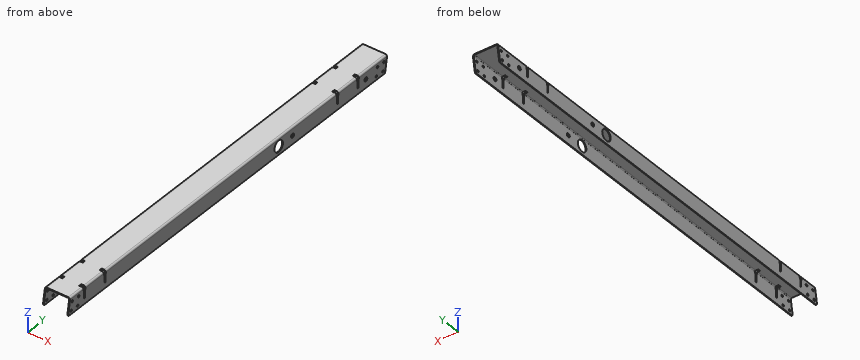
from build123d import *

# Parameters (mm, degrees)
SKETCH1_W                        = 57.15
SKETCH1_H                        = 946.658
BASE_FLANGE1_DEPTH               = 1.89738
EDGE_FLANGE1_STRIP_W             = 11.65352
EDGE_FLANGE1_STRIP_H             = 1.89738
EDGE_FLANGE1_STRIP_CUT_DEPTH     = 946.658
EDGE_FLANGE1_DEPTH               = 946.658
EDGE_FLANGE1_FLAT_DEPTH          = 1.89738
EDGE_FLANGE2_STRIP_W             = 11.65352
EDGE_FLANGE2_STRIP_H             = 1.89738
EDGE_FLANGE2_STRIP_CUT_DEPTH     = 946.658
EDGE_FLANGE2_DEPTH               = 946.658
EDGE_FLANGE2_FLAT_DEPTH          = 1.89738
FILLET1_R                        = 2.54
SKETCH12_R                       = 2.4638
CUT_EXTRUDE1_DEPTH               = 484.620370701
SKETCH13_R                       = 2.4638
CUT_EXTRUDE2_DEPTH               = 484.620370701
CUT_EXTRUDE3_DEPTH               = 9.525
LPATTERN1_COUNT                  = 2
LPATTERN1_PITCH                  = 755.65
MIRROR1_COPY_1_DEPTH             = 9.525
SKETCH15_R                       = 12.7
CUT_EXTRUDE4_DEPTH               = 484.620370701
F_11_32_0_34375_DIAMETER_HOLE1_D = 8.73125


# Sheet-metal steps are written as plain solids
with BuildPart() as part:
    # Sketch1 → Base-Flange1 (new body)
    with BuildSketch(Plane.XY):
        Rectangle(SKETCH1_W, SKETCH1_H)
    extrude(amount=-BASE_FLANGE1_DEPTH)

    # Edge-Flange1 strip (across the edge) → Edge-Flange1 strip cut (cut)
    with BuildSketch(Plane(origin=(28.575, 473.329, -1.89738), x_dir=(-1, 0, 0), z_dir=(0, -1, 0))):
        with Locations((-1.89738, -0.94869)):
            Rectangle(EDGE_FLANGE1_STRIP_W, EDGE_FLANGE1_STRIP_H)
    extrude(amount=EDGE_FLANGE1_STRIP_CUT_DEPTH, mode=Mode.SUBTRACT)

    # Edge-Flange1 bend section (across the edge) → Edge-Flange1 (add)
    with BuildSketch(Plane(origin=(28.575, 473.329, -1.89738), x_dir=(-1, 0, 0), z_dir=(0, -1, 0))):
        with BuildLine():
            Line((0, 2.032), (1.89738, 2.032))
            ThreePointArc((1.89738, 2.032), (2.492539021, 0.595159021), (3.92938, 0))
            Line((3.92938, 0), (3.92938, -1.89738))
            ThreePointArc((3.92938, -1.89738), (1.150888756, -0.746491244), (0, 2.032))
        make_face()
    extrude(amount=EDGE_FLANGE1_DEPTH)

    # Edge-Flange1 profile (on flange) → Edge-Flange1 flat (add)
    with BuildSketch(Plane(origin=(28.575, 0, -1.89738), x_dir=(0, 1, 0), z_dir=(-1, 0, 0))):
        Polygon((473.329, 2.032), (473.329, 2.87782), (467.452938633, 36.20262), (-479.205061367, 36.20262), (-473.329, 2.87782), (-473.329, 2.032), align=None)
    extrude(amount=EDGE_FLANGE1_FLAT_DEPTH)

    # Edge-Flange2 strip (across the edge) → Edge-Flange2 strip cut (cut)
    with BuildSketch(Plane(origin=(-28.575, -473.329, -1.89738), x_dir=(1, 0, 0), z_dir=(0, 1, 0))):
        with Locations((-1.89738, -0.94869)):
            Rectangle(EDGE_FLANGE2_STRIP_W, EDGE_FLANGE2_STRIP_H)
    extrude(amount=EDGE_FLANGE2_STRIP_CUT_DEPTH, mode=Mode.SUBTRACT)

    # Edge-Flange2 bend section (across the edge) → Edge-Flange2 (add)
    with BuildSketch(Plane(origin=(-28.575, -473.329, -1.89738), x_dir=(1, 0, 0), z_dir=(0, 1, 0))):
        with BuildLine():
            Line((0, 2.032), (1.89738, 2.032))
            ThreePointArc((1.89738, 2.032), (2.492539021, 0.595159021), (3.92938, 0))
            Line((3.92938, 0), (3.92938, -1.89738))
            ThreePointArc((3.92938, -1.89738), (1.150888756, -0.746491244), (0, 2.032))
        make_face()
    extrude(amount=EDGE_FLANGE2_DEPTH)

    # Edge-Flange2 profile (on flange) → Edge-Flange2 flat (add)
    with BuildSketch(Plane(origin=(-28.575, 0, -1.89738), x_dir=(0, -1, 0), z_dir=(1, 0, 0))):
        Polygon((-473.329, 2.87782), (-473.329, 2.032), (473.329, 2.032), (473.329, 2.87782), (479.205061367, 36.20262), (-467.452938633, 36.20262), align=None)
    extrude(amount=EDGE_FLANGE2_FLAT_DEPTH)

    # Fillet1
    fillet1_edges = [part.edges().sort_by_distance(p)[0] for p in [
        (27.62631, -479.205061367, -38.1),
        (27.62631, 467.452938633, -38.1),
        (-27.62631, 467.452938633, -38.1),
        (-27.62631, -479.205061367, -38.1),
    ]]
    fillet(fillet1_edges, radius=FILLET1_R)

    # Sketch12 → Cut-Extrude1 (cut, through all)
    with BuildSketch(Plane.ZY.offset(28.575)):
        with Locations((-30.48, -470.123898991)):
            Circle(SKETCH12_R)
        with Locations((-30.48, -450.780022035)):
            Circle(SKETCH12_R)
        with Locations((-11.43, -447.420993052)):
            Circle(SKETCH12_R)
        with Locations((-11.43, -466.764870009)):
            Circle(SKETCH12_R)
    extrude(amount=-CUT_EXTRUDE1_DEPTH, mode=Mode.SUBTRACT)

    # Sketch13 → Cut-Extrude2 (cut, through all)
    with BuildSketch(Plane.ZY.offset(28.575)):
        with Locations((-30.48, 461.058999444)):
            Circle(SKETCH13_R)
        with Locations((-11.43, 464.418028426)):
            Circle(SKETCH13_R)
        with Locations((-11.43, 445.07415147)):
            Circle(SKETCH13_R)
        with Locations((-30.48, 441.715122487)):
            Circle(SKETCH13_R)
    extrude(amount=-CUT_EXTRUDE2_DEPTH, mode=Mode.SUBTRACT)

    # Sketch14 → Cut-Extrude3 (cut)
    with BuildSketch(Plane.ZY.offset(28.575)):
        Polygon((3.175, 389.509), (3.175, 383.159), (-5.08, 383.159), (-10.16, 385.064), (-25.4, 385.064), (-25.4, 387.604), (-10.16, 387.604), (-5.08, 389.509), align=None)
        Polygon((3.175, 328.549), (3.175, 322.199), (-5.08, 322.199), (-10.16, 324.104), (-25.4, 324.104), (-25.4, 326.644), (-10.16, 326.644), (-5.08, 328.549), align=None)
    cut_extrude3 = extrude(amount=-CUT_EXTRUDE3_DEPTH, mode=Mode.SUBTRACT)

    # LPattern1: Cut-Extrude3 ×2
    with Locations(*[(0, -i * LPATTERN1_PITCH, 0) for i in range(1, LPATTERN1_COUNT)]):
        add(cut_extrude3, mode=Mode.SUBTRACT)

    # Mirror1: Cut-Extrude3 across plane
    add(cut_extrude3.mirror(Plane(origin=(0, 0, 0), x_dir=(0, 0, 1), z_dir=(1, 0, 0))), mode=Mode.SUBTRACT)

    # Mirror1 copy 1 sketch → Mirror1 copy 1 (cut)
    with BuildSketch(Plane(origin=(28.575, -755.65, 0), x_dir=(0, 0, 1), z_dir=(1, 0, 0))):
        Polygon((3.175, -389.509), (3.175, -383.159), (-5.08, -383.159), (-10.16, -385.064), (-25.4, -385.064), (-25.4, -387.604), (-10.16, -387.604), (-5.08, -389.509), align=None)
        Polygon((3.175, -328.549), (3.175, -322.199), (-5.08, -322.199), (-10.16, -324.104), (-25.4, -324.104), (-25.4, -326.644), (-10.16, -326.644), (-5.08, -328.549), align=None)
    extrude(amount=-MIRROR1_COPY_1_DEPTH, mode=Mode.SUBTRACT)

    # Sketch15 → Cut-Extrude4 (cut, through all)
    with BuildSketch(Plane.ZY.offset(28.575)):
        with Locations((-19.05, 149.961528499)):
            Circle(SKETCH15_R)
    extrude(amount=-CUT_EXTRUDE4_DEPTH, mode=Mode.SUBTRACT)

    # 11/32 (0.34375) Diameter Hole1 (through all)
    with Locations(Plane.ZY.offset(28.575)):
        with Locations((-19.05, 410.201153152), (-19.05, 191.126153152)):
            Hole(F_11_32_0_34375_DIAMETER_HOLE1_D / 2)


solid = part.part
For this review, take the finished solid that the model builds, in its own axes (mm). Round coordinates to 2 decimals unless told otherwise and drop trailing zeros. Loops run counter-clockwise (first coordinate to the right, second up) from the corner with the lowest first, then second, coordinate; pieces in that order, holes last. Notation, with made-up numbers: (-2, 28.25) - (47, 28.25) arc R14 cw to (47, 37.25) - close; hole circle Ø1 at (-10, 75). An arc over 180 degrees is marked (long way). Answer as CSV lines item,"result".
(1) Wall thickness on line 1 (X direction, y = -238.5, z = -5.5) (3 decimals); line 2 (Y direction, x = -27, z = -30); line 3 (Z direction, x = -3, y = 368): over which ranges is each line inside the solid? List them lowest first.
Checked values:
line 1,"x = -28.575 to -26.678, 26.678 to 28.575"
line 2,"y = -477.78 to -472.54, -467.71 to -453.2, -448.36 to 143.53, 156.39 to 439.3, 444.13 to 458.64, 463.48 to 468.88"
line 3,"z = -1.9 to 0"
(2) Insertion check: P1, Ø2, axis at x = 27.5, z = -15.5, coming from the -Y side; P2, Ø6, axis at x = 20, y = -223.5, coming from the -Z side; P3, Ø4.5, axis at y = 461.059, z = -30.48, coming from the +X side; P4, Ø5.5, axis at x = -22.5, z = -3.5, coming from the -Y side. Each pin has a flat end and moves straight along its axis. Give the tip position at first contact, or say it passes through.
Checked values:
P1,"stops at y = -475.4"
P2,"stops at z = -1.9"
P3,"passes through"
P4,"stops at y = -473.33"
(3) Consider section B-B on x = -4. Give the boundary of the cut face in (y, z).
Checked values:
outline,"(-473.33, -1.9) - (473.33, -1.9) - (473.33, 0) - (-473.33, 0) - close"
(4) Consider section A-A on y = 1. Give the boundary of the cut face in (x, z) (3 decimals), then the cut area to 3 significant figures.
Checked values:
outline,"(-28.575, -38.1) - (-26.678, -38.1) - (-26.678, -3.929) arc R2.032 cw to (-24.646, -1.897) - (24.646, -1.897) arc R2.032 cw to (26.678, -3.929) - (26.678, -38.1) - (28.575, -38.1) - (28.575, -3.929) arc R3.929 ccw to (24.646, 0) - (-24.646, 0) arc R3.929 ccw to (-28.575, -3.929) - close"
area,"241 mm2"
